Autodesk Inventor part; units mm, degrees
ref_plane "Mirror plane" through (14.9666, -47.2893, -153.2107) normal (0, 0, -1) x (-1, 0, 0)
ref_plane "Mirror plane 2" through (0, -46.2893, -160.7107) normal (0, 0, -1) x (-1, 0, 0)
ref_plane "YZ Plane" through (0, 0, 0) normal (1, 0, 0) x (0, 1, 0)
sketch "Sketch2" plane through (0, 0, 0) normal (1, 0, 0) x (0, 1, 0)
  line L0 (0, 0) -> (0, -50)
  arc A0 (-14.6447, -85.3553) -> (0, -50) centre (-50, -50) ccw
  line L1 (-50, -50) -> (-14.6447, -85.3553) construction
  line L2 (-50, -50) -> (0, -50) construction
  arc A1 (-14.6447, -85.3553) -> (-29.2893, -120.7107) centre (20.7107, -120.7107) ccw
  line L3 (20.7107, -120.7107) -> (-29.2893, -120.7107) construction
  line L4 (20.7107, -120.7107) -> (-14.6447, -85.3553) construction
  line L5 (-29.2893, -120.7107) -> (-29.2893, -140.7107)
  line L6 (0, 0) -> (-92.5786, 0) construction
  line L7 (-2, 0) -> (-2, -50)
  arc A2 (-16.6447, -85.3553) -> (-2, -50) centre (-52, -50) ccw
  arc A3 (-16.6447, -85.3553) -> (-31.2893, -120.7107) centre (18.7107, -120.7107) ccw
  line L8 (-31.2893, -120.7107) -> (-31.2893, -140.7107)
  line L9 (0, 0) -> (-2, 0)
  line L10 (-29.2893, -140.7107) -> (-31.2893, -140.7107)
  line L11 (-46.2893, -140.7107) -> (-46.2893, 0)
  line L12 (-31.2893, -140.7107) -> (-46.2893, -140.7107) construction
  dimension "d18" = 50
  dimension "d19" = 45
  dimension "d20" = 45
  dimension "d21" = 50
  dimension "d22" = 50
  dimension "d23" = 20
  dimension "d26" = 2
  dimension "d31" = 90
  dimension "d32" = 15
revolve "Revolution1" add sketch "Sketch2" angle 360 about axis through (0, -46.2893, -140.7107) along (0, 0, 1)
sketch "Sketch3" plane through (0, -46.2893, -140.7107) normal (0, 0, -1) x (-1, 0, 0)
  circle A0 centre (0, 0) radius 15
  circle A1 centre (0, 0) radius 2
  circle A2 centre (0, 0) radius 4
  point P0 (0, 46.2893)
  dimension "d34" = 4
  dimension "d35" = 8
extrude "Extrusion1" add sketch "Sketch3" against normal blind 10 contours A2
sketch "Sketch4" plane through (0, -46.2893, -140.7107) normal (0, 0, -1) x (-1, 0, 0)
  circle A0 centre (0, 0) radius 15
  circle A1 centre (0, 0) radius 4
  line L0 (-3.873, -1) -> (-14.9666, -1)
  line L1 (-3.873, 1) -> (-14.9666, 1)
  circle A2 centre (0, 0) radius 15
  line L2 (-4, 0) -> (-15, 0) construction
  line L3 (64.8051, 46.2893) -> (-64.8051, 46.2893)
  point P0 (0, 46.2893)
  dimension "d38" = 0
  dimension "d39" = 1
  dimension "d40" = 1
extrude "Extrusion2" add sketch "Sketch4" against normal blind 4 contours L1 A1 L0 A0 picked at (-7.656, -0.1112)
pattern_circular "Circular Pattern1" count 5 over 360 about axis through (0, -46.2893, -140.7107) along (0, 0, 1) of "Extrusion2"
sketch "Sketch5" plane through (0, -46.2893, -140.7107) normal (0, 0, -1) x (-1, 0, 0)
  circle A0 centre (0, 0) radius 17
  circle A1 centre (0, 0) radius 15
  point P0 (0, 46.2893)
  dimension "d46" = 30
extrude "Extrusion3" add sketch "Sketch5" along normal blind 15
sketch "Sketch6" plane through (0, -46.2893, -155.7107) normal (0, 0, -1) x (-1, 0, 0)
  circle A0 centre (0, 0) radius 17
  circle A1 centre (0, 0) radius 23
  point P0 (0, 46.2893)
  dimension "d49" = 46
extrude "Extrusion4" add sketch "Sketch6" against normal blind 4
sketch "Sketch7" plane through (0, -46.2893, -155.7107) normal (0, 0, -1) x (-1, 0, 0)
  circle A0 centre (0, 0) radius 23
  circle A1 centre (0, 0) radius 21
  point P0 (0, 46.2893)
  dimension "d52" = 42
extrude "Extrusion5" add sketch "Sketch7" along normal blind 10
sketch "Sketch8" plane through (0, -46.2893, -165.7107) normal (0, 0, -1) x (-1, 0, 0)
  circle A0 centre (0, 0) radius 21
  circle A1 centre (0, 0) radius 23
  circle A2 centre (0, 0) radius 23
  line L0 (0, -23) -> (0, -21)
  line L1 (23, 0) -> (21, 0)
  line L2 (64.8051, 46.2893) -> (-64.8051, 46.2893)
  line L3 (0, -64.8051) -> (0, 64.8051)
  point P0 (0, 46.2893)
  dimension "d55" = 2
  dimension "d56" = 2
extrude "Extrusion6" cut sketch "Sketch8" against normal blind 10 contours A0 L1 A1 L0
ref_plane "Mirror plane" through (14.9666, -47.2893, -153.2107) normal (0, 0, -1) x (-1, 0, 0)
mirror "Mirror1" about plane through (14.9666, -47.2893, -153.2107) normal (0, 0, -1) of "Extrusion2", "Circular Pattern1", "Extrusion1"
ref_plane "Mirror plane 2" through (0, -46.2893, -160.7107) normal (0, 0, -1) x (-1, 0, 0)
mirror "Mirror2" about plane through (0, -46.2893, -160.7107) normal (0, 0, -1) of "Extrusion4", "Extrusion3"
equation "\"d40\" = d39"
properties part number "Outer tube"
Build history of the part. All positions in model axes, mm. A direction names the side the tool comes from. Coordinates: 2 decimals unless noted, no trailing zeros. Order: outer loops, then holes, each group sorted by start corner. A loop starts at its lowest first (then second) coordinate and runs counter-clockwise, first axis right, second up. Notation, with made-up numbers: (23.5, 28) - (71.5, 28) arc R25 ccw to (71.5, 60) - close; hole circle Ø10 at (0.25, 24.5). An arc over 180 degrees is marked (long way). Put each result on its own line as item: value.
1. Tool access for faces 1 (the face through (15.331, -31.938, -160.641)), 2 (the face through (-3.815, -45.088, -134.67)), 3 (the face through (1, -44, -175.711)), 4 (the face through (3.886, -37.566, -167.683)): list every direction of +Z, -Z, +X, -X, +Y, -Y with a clear straight run to the whole face (end or side of a thin tool).
Answer sheet:
face 1: none
face 2: +Z
face 3: -Z
face 4: +Z, -Z
2. Probe line 1 along Y through (x, z) = (0, -135); line 2 along Y through (x, z) = (0, -26); line 3 along Z through (x, y) = (-20.5, -53.5). List the from-to ranges inside material, lowest first. Write a range as [from, to].
Answer sheet:
line 1: y = [-63.29, -61.29], [-50.29, -48.29], [-44.29, -42.29], [-31.29, -29.29]
line 2: y = [-92.58, -90.58], [-2, 0]
line 3: z = [-169.71, -165.71], [-155.71, -151.71], [-99.48, -95.65]
3. Pull direction X, two halves, no side cores. Call faces 5 (the face through (10, -58, -180.711)), 6 (the face through (1.936, -55.483, -138.739)), 7 (the face through (18.25, -32.29, -160.58)): pulls with the +X half, pulls with the -X half, needs draft (parallel to the pull), parting line crosses it, or undercut.
Answer sheet:
face 5: needs draft
face 6: undercut
face 7: parting line crosses it
4. Saw through at A-A (z = -158). Write the cut outline in (x, y).
Answer sheet:
outline: (-23, -46.29) - (-21, -46.29) arc R21 cw (long way) to (0, -67.29) - (0, -69.29) arc R23 ccw (long way) to start
5. Drop flat-ended pins along their axis: P1, Ø5, axis at x = 0, y = -46.29, coming from the -Z side; P2, Ø1, axis at y = -18.5, z = -76.5, coming from the -X side; P3, Ø1.6, axis at x = 3.5, y = -35, coming from the -Z side; P4, Ø9, axis at x = -10, y = -39, coming from the -Z side. Give the stop position or say it passes through.
Answer sheet:
P1: stops at z = -175.71
P2: stops at x = -27.59
P3: stops at z = -169.71
P4: stops at z = -180.71
